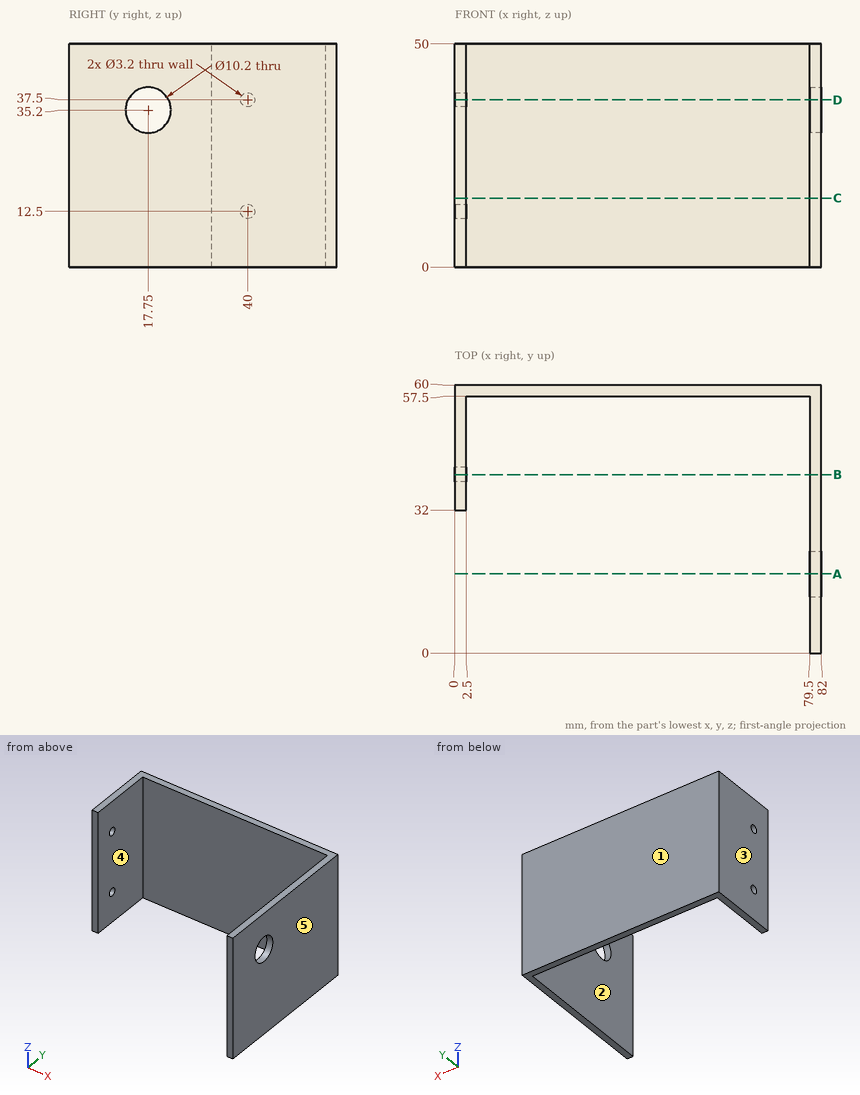
Geometry check sheet. Reference: drawing and pictorial views, mm from the part's lowest x, y, z. A direction names the side the tool comes from. Give positions to 0.01 mm unless a question says otherwise; leave off trailing zeros. Order: outer loops, then holes, each group sorted by start corner. A loop starts at its lowest first (then second) coordinate and runs counter-clockwise, first axis right, second up. Notation, with made-up numbers: M -24.75,-29.75 L -15.75,-29.75 A21 cw -15.75,7.25 Z; hole C 15.25,65 d11. An arc over 180 degrees is marked long. Return JSON: item names as keys, results as strings. Group by question number.
1) Scan lines: line 1 (Y direction, x = 81.35, z = 35.2); line 2 (X direction, y = 39, z = 10); line 3 (Y direction, x = 1.3, z = 12.5). Record each from-to range of solid material in increasing order.
2) Section check B-B on y = 40. Record the cut outline in (x, z).
3) Access from +Z, -Z, +X, -X, +Y, -Y to the whole of each face (thin tool, end or side, straight path). Record for the marked faces 4 and 5.
4) Section check D-D on z = 37.5. Record the cut outline in (x, y).
5) Section check C-C on z = 15.5. Record the cut outline in (x, y), and give its area (4 significant figures).
6) Go/stop test with flat-tipped pins: pin 1 Ø3 at (x, z) = (22, 15) entering from -Y; pin 2 Ø25 at (y, z) = (29, 15.5) entering from -X; pin 3 Ø3 at (y, z) = (8, 21) entering from -X; pin 4 Ø8 at (y, z) = (17.75, 35.2) entering from +X. Record where each tip stops, or that it passes through.
7) Section check A-A on y = 17.75. Record the cut outline in (x, z).
8) Mould release check, pull along X, two halves, no side actions. Record for the marked faces 1, 2 and 3: pulls with the +X half, pulls with the -X half, needs draft (parallel to the pull), parting line crosses it, or undercut.
Answer block:
{
 "1": {"line 1": "y = 0 to 12.65, 22.85 to 60", "line 2": "x = 0 to 2.5, 79.5 to 82", "line 3": "y = 32 to 38.4, 41.6 to 60"},
 "2": {"outline": "M 0,0 L 2.5,0 L 2.5,10.9 L 0,10.9 Z; M 0,14.1 L 2.5,14.1 L 2.5,35.9 L 0,35.9 Z; M 0,39.1 L 2.5,39.1 L 2.5,50 L 0,50 Z; M 79.5,0 L 82,0 L 82,50 L 79.5,50 Z"},
 "3": {"face 4": "+Z, -Z, -Y", "face 5": "+Z, -Z, +X, +Y, -Y"},
 "4": {"outline": "M 0,32 L 2.5,32 L 2.5,38.4 L 0,38.4 Z; M 0,41.6 L 2.5,41.6 L 2.5,57.5 L 79.5,57.5 L 79.5,22.3 L 82,22.3 L 82,60 L 0,60 Z; M 79.5,0 L 82,0 L 82,13.2 L 79.5,13.2 Z"},
 "5": {"outline": "M 0,32 L 2.5,32 L 2.5,57.5 L 79.5,57.5 L 79.5,0 L 82,0 L 82,60 L 0,60 Z", "area": "412.5 mm^2"},
 "6": {"pin 1": "stops at y = 57.5", "pin 2": "stops at x = 0", "pin 3": "stops at x = 79.5", "pin 4": "passes through"},
 "7": {"outline": "M 79.5,0 L 82,0 L 82,30.1 L 79.5,30.1 Z; M 79.5,40.3 L 82,40.3 L 82,50 L 79.5,50 Z"},
 "8": {"face 1": "needs draft", "face 2": "undercut", "face 3": "pulls with the -X half"}
}
